Input: dimensioned drawing with shaded views. Units: mm. Origin: part minimum x, y, z. A direction names the side the tool comes from. Round coordinates to 2 decimals unless told otherwise and drop trailing zeros. Loops run counter-clockwise (first coordinate to the right, second up) from the corner with the lowest first, then second, coordinate; pieces in that order, holes last. Notation, with made-up numbers: M 63,-22.5 L 77,-22.5 A19 ccw 77,6.5 Z; hole C 14.25,36 d9. An arc over 180 degrees is marked long. Use one line per item in the form item = value. Start each with the question number.
Q1. Section query B-B, the plane y = 23.75. Output: boundary loops of the cut face in (x, z) (3 decimals).
Q2. Ray query, line 1 along Z through (x, y) = (21, 17.25) (3 decimals); line 2 along Y through (x, z) = (25.5, 48); line 3 along X through (y, z) = (9.5, 95) (3 decimals). Return the intervals inside material, ascending.
Q3. Section query C-C, the plane z = 15. Output: boundary loops of the cut face in (x, y) (3 decimals), and give its area (3 significant figures).
Q4. First-contact query: P1, Ø5.5, axis at x = 8.5, y = 16, coming from the -Z side (3 decimals); P2, Ø1.9, axis at y = 9.5, z = 67, coming from the -X side (3 decimals); P3, Ø3.5, axis at y = 16.5, z = 28, coming from the +X side (3 decimals). Flat tips, straight axial feed; report the tip coordinate or a pass-through.
Q5. Section query D-D, the plane x = 21. Output: boundary loops of the cut face in (y, z) (3 decimals).
Q6. Access query for the marked faces 1 and 2. Directions: +Z, -Z, +X, -X, +Y, -Y. A direction counts if a zero-diameter tool reaches every point of the face in a straight line with its end or side. Return the directions, or none.
Q7. Section query A-A, the plane y = 8. Output: boundary loops of the cut face in (x, z) (3 decimals).
Q8. Mould query, pull axis Z, two halves, no side actions, for the marked faces 3, 4, 5 and 6. Classes: pulls with the +Z half, pulls with the -Z half, needs draft (parallel to the pull), parting line crosses it, or undercut.
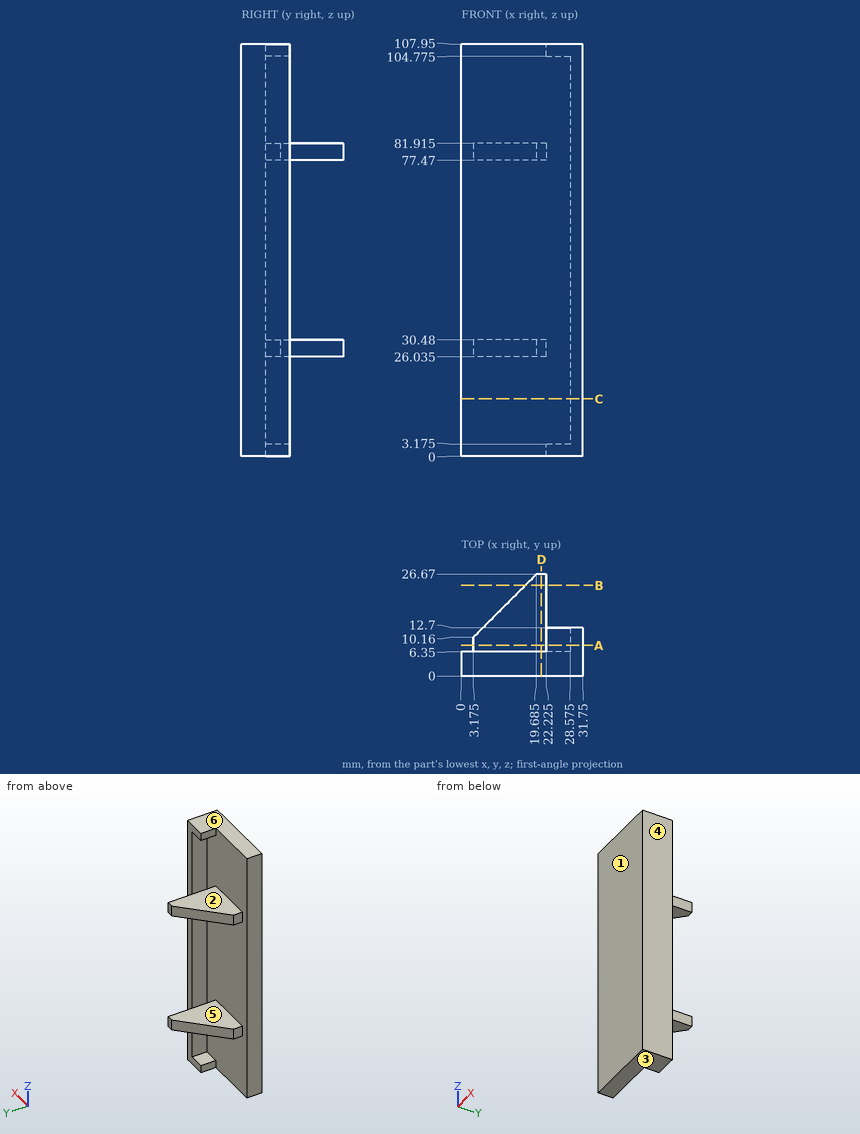
Results found:
q1.outline = M 16.765,26.035 L 22.225,26.035 L 22.225,30.48 L 16.765,30.48 Z; M 16.765,77.47 L 22.225,77.47 L 22.225,81.915 L 16.765,81.915 Z
q2.line_1 = 26.035 to 30.48, 77.47 to 81.915
q2.line_2 = 0 to 6.35
q2.line_3 = 28.575 to 31.75
q3.outline = M 0,0 L 31.75,0 L 31.75,12.7 L 28.575,12.7 L 28.575,6.35 L 0,6.35 Z
q3.area = 222 mm²
q4.P1 = 26.035
q4.P2 = 28.575
q4.P3 = 22.225
q5.outline = M 0,0 L 6.35,0 L 6.35,26.035 L 26.67,26.035 L 26.67,30.48 L 6.35,30.48 L 6.35,77.47 L 26.67,77.47 L 26.67,81.915 L 6.35,81.915 L 6.35,107.95 L 0,107.95 Z
q6.face_1 = +Z, -Z, +X, -X, -Y
q6.face_2 = +Z, -X, +Y
q7.outline = M 3.175,26.035 L 22.225,26.035 L 22.225,30.48 L 3.175,30.48 Z; M 3.175,77.47 L 22.225,77.47 L 22.225,81.915 L 3.175,81.915 Z; M 22.225,0 L 31.75,0 L 31.75,107.95 L 22.225,107.95 L 22.225,104.775 L 28.575,104.775 L 28.575,3.175 L 22.225,3.175 Z
q8.face_3 = pulls with the -Z half
q8.face_4 = needs draft
q8.face_5 = undercut
q8.face_6 = pulls with the +Z half
